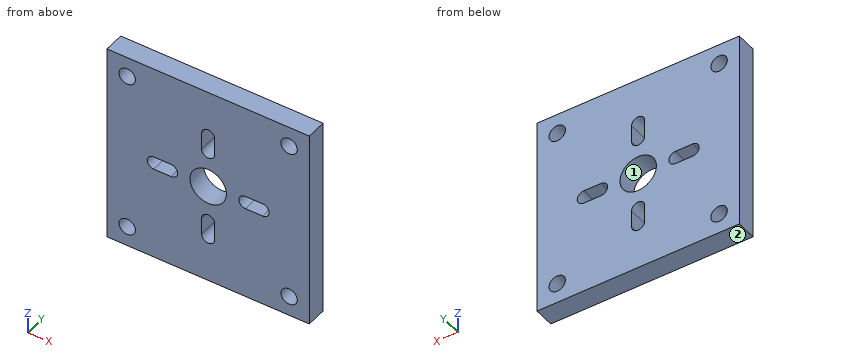
```python
from build123d import *

# Parameters (mm, degrees)
SKETCH1_W          = 100
SKETCH1_H          = 100
BASE_DEPTH         = 10
SKETCH2_R          = 9
ACTUATOR_CUT_DEPTH = 40
CUT_EXTRUDE1_REACH = 73.414
CUT_EXTRUDE2_REACH = 73.414
SKETCH5_R          = 4.05


with BuildPart() as part:
    # Sketch1 → base (new body)
    with BuildSketch(Plane(origin=(0, 0, 0), x_dir=(1, 0, 0), z_dir=(0, 1, 0))):
        Rectangle(SKETCH1_W, SKETCH1_H)
    extrude(amount=BASE_DEPTH)

    # Sketch2 → actuator cut (cut)
    with BuildSketch(Plane(origin=(0, 10, 0), x_dir=(1, 0, 0), z_dir=(0, 1, 0))):
        with Locations(Location((0, 0, 0), (0, 0, 270))):
            Circle(SKETCH2_R)
    extrude(amount=-ACTUATOR_CUT_DEPTH, mode=Mode.SUBTRACT)

    # Sketch3 → Cut-Extrude1 (cut, up to next)
    with BuildSketch(Plane(origin=(0, 10, 0), x_dir=(1, 0, 0), z_dir=(0, 1, 0)), mode=Mode.PRIVATE) as cut_extrude1_sk1:
        with BuildLine():
            Line((3.25, -26.870057685), (3.25, -18.384776311))
            ThreePointArc((3.25, -18.384776311), (0, -15.134776311), (-3.25, -18.384776311))
            Line((-3.25, -18.384776311), (-3.25, -26.870057685))
            ThreePointArc((-3.25, -26.870057685), (0, -30.120057685), (3.25, -26.870057685))
        make_face()
    cut_extrude1_tool1 = extrude(cut_extrude1_sk1.sketch, amount=-CUT_EXTRUDE1_REACH, mode=Mode.PRIVATE) & part.part
    # Sketch3 → Cut-Extrude1 (cut, up to next)
    with BuildSketch(Plane(origin=(0, 10, 0), x_dir=(1, 0, 0), z_dir=(0, 1, 0)), mode=Mode.PRIVATE) as cut_extrude1_sk2:
        with BuildLine():
            Line((26.870057685, 3.25), (18.384776311, 3.25))
            ThreePointArc((18.384776311, 3.25), (15.134776311, 0), (18.384776311, -3.25))
            Line((18.384776311, -3.25), (26.870057685, -3.25))
            ThreePointArc((26.870057685, -3.25), (30.120057685, 0), (26.870057685, 3.25))
        make_face()
    cut_extrude1_tool2 = extrude(cut_extrude1_sk2.sketch, amount=-CUT_EXTRUDE1_REACH, mode=Mode.PRIVATE) & part.part
    # Sketch3 → Cut-Extrude1 (cut, up to next)
    with BuildSketch(Plane(origin=(0, 10, 0), x_dir=(1, 0, 0), z_dir=(0, 1, 0)), mode=Mode.PRIVATE) as cut_extrude1_sk3:
        with BuildLine():
            Line((-26.870057685, -3.25), (-18.384776311, -3.25))
            ThreePointArc((-18.384776311, -3.25), (-15.134776311, 0), (-18.384776311, 3.25))
            Line((-18.384776311, 3.25), (-26.870057685, 3.25))
            ThreePointArc((-26.870057685, 3.25), (-30.120057685, 0), (-26.870057685, -3.25))
        make_face()
    cut_extrude1_tool3 = extrude(cut_extrude1_sk3.sketch, amount=-CUT_EXTRUDE1_REACH, mode=Mode.PRIVATE) & part.part
    # Sketch3 → Cut-Extrude1 (cut, up to next)
    with BuildSketch(Plane(origin=(0, 10, 0), x_dir=(1, 0, 0), z_dir=(0, 1, 0)), mode=Mode.PRIVATE) as cut_extrude1_sk4:
        with BuildLine():
            Line((-3.25, 26.870057685), (-3.25, 18.384776311))
            ThreePointArc((-3.25, 18.384776311), (0, 15.134776311), (3.25, 18.384776311))
            Line((3.25, 18.384776311), (3.25, 26.870057685))
            ThreePointArc((3.25, 26.870057685), (0, 30.120057685), (-3.25, 26.870057685))
        make_face()
    cut_extrude1_tool4 = extrude(cut_extrude1_sk4.sketch, amount=-CUT_EXTRUDE1_REACH, mode=Mode.PRIVATE) & part.part
    add(cut_extrude1_tool1.solids().sort_by_distance((0, 10, 22.627417))[0], mode=Mode.SUBTRACT)
    add(cut_extrude1_tool2.solids().sort_by_distance((22.627417, 10, 0))[0], mode=Mode.SUBTRACT)
    add(cut_extrude1_tool3.solids().sort_by_distance((-22.627417, 10, 0))[0], mode=Mode.SUBTRACT)
    add(cut_extrude1_tool4.solids().sort_by_distance((0, 10, -22.627417))[0], mode=Mode.SUBTRACT)

    # Sketch5 → Cut-Extrude2 (cut, up to next)
    with BuildSketch(Plane(origin=(0, 10, 0), x_dir=(1, 0, 0), z_dir=(0, 1, 0)), mode=Mode.PRIVATE) as cut_extrude2_sk1:
        with Locations(Location((-40, -40, 0), (0, 0, 270))):
            Circle(SKETCH5_R)
    cut_extrude2_tool1 = extrude(cut_extrude2_sk1.sketch, amount=-CUT_EXTRUDE2_REACH, mode=Mode.PRIVATE) & part.part
    # Sketch5 → Cut-Extrude2 (cut, up to next)
    with BuildSketch(Plane(origin=(0, 10, 0), x_dir=(1, 0, 0), z_dir=(0, 1, 0)), mode=Mode.PRIVATE) as cut_extrude2_sk2:
        with Locations(Location((-40, 40, 0), (0, 0, 270))):
            Circle(SKETCH5_R)
    cut_extrude2_tool2 = extrude(cut_extrude2_sk2.sketch, amount=-CUT_EXTRUDE2_REACH, mode=Mode.PRIVATE) & part.part
    # Sketch5 → Cut-Extrude2 (cut, up to next)
    with BuildSketch(Plane(origin=(0, 10, 0), x_dir=(1, 0, 0), z_dir=(0, 1, 0)), mode=Mode.PRIVATE) as cut_extrude2_sk3:
        with Locations(Location((40, -40, 0), (0, 0, 270))):
            Circle(SKETCH5_R)
    cut_extrude2_tool3 = extrude(cut_extrude2_sk3.sketch, amount=-CUT_EXTRUDE2_REACH, mode=Mode.PRIVATE) & part.part
    # Sketch5 → Cut-Extrude2 (cut, up to next)
    with BuildSketch(Plane(origin=(0, 10, 0), x_dir=(1, 0, 0), z_dir=(0, 1, 0)), mode=Mode.PRIVATE) as cut_extrude2_sk4:
        with Locations(Location((40, 40, 0), (0, 0, 270))):
            Circle(SKETCH5_R)
    cut_extrude2_tool4 = extrude(cut_extrude2_sk4.sketch, amount=-CUT_EXTRUDE2_REACH, mode=Mode.PRIVATE) & part.part
    add(cut_extrude2_tool1.solids().sort_by_distance((-40, 10, 40))[0], mode=Mode.SUBTRACT)
    add(cut_extrude2_tool2.solids().sort_by_distance((-40, 10, -40))[0], mode=Mode.SUBTRACT)
    add(cut_extrude2_tool3.solids().sort_by_distance((40, 10, 40))[0], mode=Mode.SUBTRACT)
    add(cut_extrude2_tool4.solids().sort_by_distance((40, 10, -40))[0], mode=Mode.SUBTRACT)


solid = part.part
```
CAD build for the part. Positions are in the model's coordinates, mm. Face numbers are marked on the shaded views. Round coordinates to 2 decimals unless told otherwise and drop trailing zeros. Write each loop counter-clockwise with the first axis right and the second up, starting at its lowest first coordinate (ties: lowest second). Pieces come first, ordered by that corner, then holes.
Item 1: Mould opens along X. For the marked faces 1 and 2 say: released by +X, released by -X, zero draft, split by the parting line, or undercut.
Filled in:
face 1: undercut
face 2: zero draft
Item 2: Band-saw the part on C-C on y = 2.5. Give the number of separate pieces and of enclosed holes in the cut face, then the cut area to 3 significant figures.
Filled in:
separate pieces: 1
enclosed holes: 9
area: 9,190 mm2
Item 3: Band-saw the part on B-B on z = 0. Write the cut outline in (x, y).
Filled in:
outline: (-50, 0) - (-30.12, 0) - (-30.12, 10) - (-50, 10) - close; (-15.13, 0) - (-9, 0) - (-9, 10) - (-15.13, 10) - close; (9, 0) - (15.13, 0) - (15.13, 10) - (9, 10) - close; (30.12, 0) - (50, 0) - (50, 10) - (30.12, 10) - close
Item 4: Band-saw the part on A-A on x = 40. Write the cut outline in (y, z), then the cut area to 3 significant figures.
Filled in:
outline: (0, -50) - (10, -50) - (10, -44.05) - (0, -44.05) - close; (0, -35.95) - (10, -35.95) - (10, 35.95) - (0, 35.95) - close; (0, 44.05) - (10, 44.05) - (10, 50) - (0, 50) - close
area: 838 mm2
Item 5: Band-saw the part on D-D on z = -40. Write the cut outline in (x, y).
Filled in:
outline: (-50, 0) - (-44.05, 0) - (-44.05, 10) - (-50, 10) - close; (-35.95, 0) - (35.95, 0) - (35.95, 10) - (-35.95, 10) - close; (44.05, 0) - (50, 0) - (50, 10) - (44.05, 10) - close
Item 6: Drill centre lines: L1, parallel to X at y = 7.25, z = 0; L2, parallel to X at y = 5, z = -40; L3, parallel to Z at x = 43, y = 2.75. Where is each one in solid material? Low to high.
Filled in:
L1: x = -50 to -30.12, -15.13 to -9, 9 to 15.13, 30.12 to 50
L2: x = -50 to -44.05, -35.95 to 35.95, 44.05 to 50
L3: z = -50 to -42.72, -37.28 to 37.28, 42.72 to 50
